Job drawing, mm, ordinate dimensions from the low corner. One solid piece. A direction names the side the tool comes from. Round coordinates to 2 decimals unless told otherwise and drop trailing zeros. Loops run counter-clockwise (first coordinate to the right, second up) from the corner with the lowest first, then second, coordinate; pieces in that order, holes last.
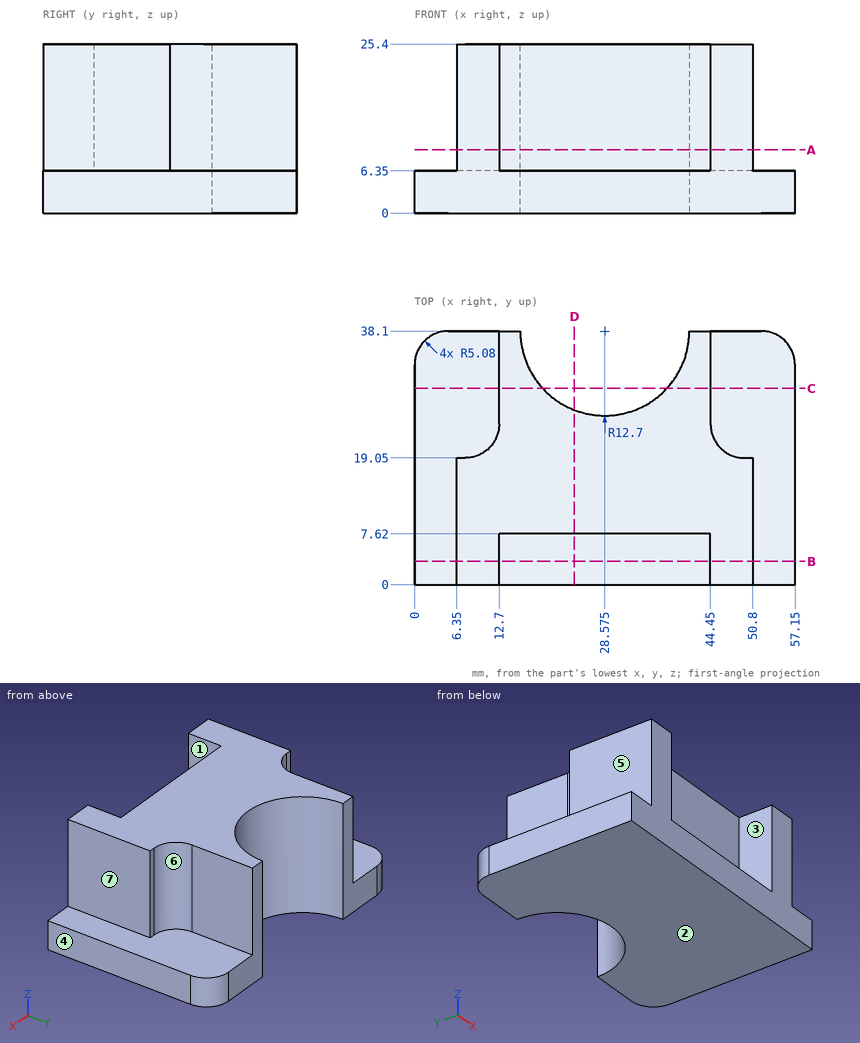
(1) Which spindle directions (+Z, -Z, +X, -X, +Y, -Y) get a long thin tool onto all of the face, cutting with end or side? Do the marked faces 5, 6 and 7. Say none if no direction does.
Responses:
face 5: +Z, -X, +Y, -Y
face 6: +Z, +X, +Y
face 7: +Z, +X, +Y, -Y
(2) Pin check, flat tips, straight feed: P1, Ø5, axis at y = 26.5, z = 19, coming from the +X side; P2, Ø1, axis at x = 7, z = 11.5, coming from the +Y side; P3, Ø7, axis at y = 29.5, z = 14.5, coming from the -X side. Stop position of each tip, or through.
Responses:
P1: stops at x = 44.45
P2: stops at y = 19.05
P3: stops at x = 12.7
(3) Slice it at B-B on y = 3.5. List the corners of the cut face in (x, z), plus the area to 3 significant figures.
Responses:
outline: (0, 0) - (57.15, 0) - (57.15, 6.35) - (50.8, 6.35) - (50.8, 25.4) - (44.45, 25.4) - (44.45, 6.35) - (12.7, 6.35) - (12.7, 25.4) - (6.35, 25.4) - (6.35, 6.35) - (0, 6.35) - close
area: 605 mm2
(4) Slice it at A-A on z = 9.5. List the corners of the cut face in (x, y) (3 decimals), plus the area to 3 significant figures.
Responses:
outline: (6.35, 0) - (12.7, 0) - (12.7, 7.62) - (44.45, 7.62) - (44.45, 0) - (50.8, 0) - (50.8, 19.05) - (49.53, 19.05) arc R5.08 cw to (44.45, 24.13) - (44.45, 38.1) - (41.275, 38.1) arc R12.7 cw to (15.875, 38.1) - (12.7, 38.1) - (12.7, 24.13) arc R5.08 cw to (7.62, 19.05) - (6.35, 19.05) - close
area: 967 mm2
(5) Pull direction X, two halves, no side cores. Call the marked faces 1, 2, 3 and 4: +X half, -X half, draft (parallel to the pull), parting line (faces both ways), or undercut.
Responses:
face 1: undercut
face 2: draft
face 3: undercut
face 4: +X half
(6) Probe line 1 (Z direction, x = 4, y = 23.5); line 2 (X direction, y = 16, z = 12); line 3 (X direction, y = 24, z = 17.5). List the from-to ranges inside material, lowest first.
Responses:
line 1: z = 0 to 6.35
line 2: x = 6.35 to 50.8
line 3: x = 12.7 to 44.45
(7) Slice it at D-D on x = 24. List the corners of the cut face in (y, z), plus the area to 3 significant figures.
Responses:
outline: (0, 0) - (26.25, 0) - (26.25, 25.4) - (7.62, 25.4) - (7.62, 6.35) - (0, 6.35) - close
area: 522 mm2
(8) Slice it at C-C on y = 29.5. List the corners of the cut face in (x, z), plus the area to 3 significant figures.
Responses:
outline: (0, 0) - (19.23, 0) - (19.23, 25.4) - (12.7, 25.4) - (12.7, 6.35) - (0, 6.35) - close; (37.92, 0) - (57.15, 0) - (57.15, 6.35) - (44.45, 6.35) - (44.45, 25.4) - (37.92, 25.4) - close
area: 493 mm2
